Geometry check sheet. Reference: the model listing, model coordinates, mm. A direction names the side the tool comes from. Give positions to 0.01 mm unless a question says otherwise; leave off trailing zeros. Write each loop counter-clockwise with the first axis right and the second up, starting at its lowest first coordinate (ties: lowest second). Pieces come first, ordered by that corner, then holes. Notation, with made-up numbers: M 18,-19.75 L 73,-19.75 A20 ccw 73,7.25 Z; hole C 69,44 d7. An arc over 180 degrees is marked long. Write each question's results on one line, items separated by ' | '.
```python
from build123d import *

# Parameters (mm, degrees)
SKETCH1_W           = 64
SKETCH1_H           = 45
BOSS_EXTRUDE1_DEPTH = 34
SKETCH2_R           = 10.75
CUT_EXTRUDE1_DEPTH  = 6
CUT_EXTRUDE2_START  = -2
SKETCH3_W           = 60
SKETCH3_H           = 41
CUT_EXTRUDE2_DEPTH  = 27
SKETCH4_W           = 60
SKETCH4_H           = 30
CUT_EXTRUDE3_DEPTH  = 43
SKETCH5_W           = 20
SKETCH5_H           = 2
CUT_EXTRUDE4_DEPTH  = 27
BOSS_EXTRUDE2_START = 2
BOSS_EXTRUDE2_DEPTH = 5
BOSS_EXTRUDE3_START = -7
BOSS_EXTRUDE3_DEPTH = 5
SKETCH10_W          = 15.255500618
SKETCH10_H          = 37
CUT_EXTRUDE5_DEPTH  = 2


with BuildPart() as part:
    # Sketch1 → Boss-Extrude1 (new body)
    with BuildSketch(Plane.XY):
        with Locations((1.653781513, -3.994957983)):
            Rectangle(SKETCH1_W, SKETCH1_H)
    extrude(amount=BOSS_EXTRUDE1_DEPTH)

    # Sketch2 → Cut-Extrude1 (cut)
    with BuildSketch(Plane.XY.offset(34)):
        with Locations((-11.346218487, -11.494957983)):
            Circle(SKETCH2_R)
    extrude(amount=-CUT_EXTRUDE1_DEPTH, mode=Mode.SUBTRACT)

    # Sketch3 → Cut-Extrude2 (cut)
    with BuildSketch(Plane.XY.offset(34).offset(CUT_EXTRUDE2_START)):
        with Locations((1.653781513, -3.994957983)):
            Rectangle(SKETCH3_W, SKETCH3_H)
    extrude(amount=-CUT_EXTRUDE2_DEPTH, mode=Mode.SUBTRACT)

    # Sketch4 → Cut-Extrude3 (cut)
    with BuildSketch(Plane(origin=(0, 18.505042017, 0), x_dir=(1, 0, 0), z_dir=(0, 1, 0))):
        with Locations((1.653781513, -17)):
            Rectangle(SKETCH4_W, SKETCH4_H)
    extrude(amount=-CUT_EXTRUDE3_DEPTH, mode=Mode.SUBTRACT)

    # Sketch5 → Cut-Extrude4 (cut)
    with BuildSketch(Plane(origin=(0, 18.505042017, 0), x_dir=(1, 0, 0), z_dir=(0, 1, 0))):
        with Locations((-11.346218487, -33)):
            Rectangle(SKETCH5_W, SKETCH5_H)
    extrude(amount=-CUT_EXTRUDE4_DEPTH, mode=Mode.SUBTRACT)

    # Sketch7 → Boss-Extrude2 (add)
    with BuildSketch(Plane(origin=(0, 0, 0), x_dir=(0, 0, -1), z_dir=(1, 0, 0)).offset(BOSS_EXTRUDE2_START)):
        with BuildLine():
            Line((0, 7.999642933), (15, 7.999642933))
            ThreePointArc((15, 7.999642933), (25, -2.000357067), (15, -12.000357067))
            Line((15, -12.000357067), (0, -12.000357067))
            Line((0, -12.000357067), (0, 7.999642933))
        make_face()
    extrude(amount=BOSS_EXTRUDE2_DEPTH)

    # Sketch8 → Boss-Extrude3 (add)
    with BuildSketch(Plane(origin=(0, 0, 0), x_dir=(0, 0, -1), z_dir=(1, 0, 0)).offset(BOSS_EXTRUDE3_START)):
        with BuildLine():
            Line((0, -12.000357067), (0, 7.999642933))
            Line((0, 7.999642933), (15, 7.999642933))
            ThreePointArc((15, 7.999642933), (25, -2.000357067), (15, -12.000357067))
            Line((15, -12.000357067), (0, -12.000357067))
        make_face()
    extrude(amount=BOSS_EXTRUDE3_DEPTH)

    # Sketch10 → Cut-Extrude5 (cut)
    with BuildSketch(Plane.ZY.offset(30.346218487)):
        with Locations((9.627750309, 0.005042017)):
            Rectangle(SKETCH10_W, SKETCH10_H)
    extrude(amount=-CUT_EXTRUDE5_DEPTH, mode=Mode.SUBTRACT)


solid = part.part
```
Q1. Access from +Z, -Z, +X, -X, +Y, -Y to the whole of each face (thin tool, end or side, straight path). Record for faces 1 (the face through (2, -2, -13)), 2 (the face through (-21.346, 6, 33)), 3 (the face through (4, 8, -7)).
Answer key:
face 1: -Z, +Y, -Y | face 2: +Z, +Y | face 3: -Z, +X, -X, +Y
Q2. Section check B-B (x = 19). Enter the section's corners in (y, z), then the cut area to 3 significant figures.
Answer key:
outline: M -26.49,0 L 18.51,0 L 18.51,2 L -24.49,2 L -24.49,32 L 18.51,32 L 18.51,34 L -26.49,34 Z | area: 240 mm2
Q3. Release check for a two-part mould opening along Y. For faces 4 (the face through (-5, -12, -8)), 5 (the face through (-29, -18.495, 10)), 6 (the face through (-11.64, -22.24, 33.01)), 7 (the face through (31.654, -3, 17)) record: released by +Y, released by -Y, zero draft, split by the parting line, or undercut.
Answer key:
face 4: released by -Y | face 5: released by +Y | face 6: undercut | face 7: zero draft
Q4. Depth check by flat-ended pin: P1, Ø15, axis at x = -9, z = 14, coming from the +Y side; P2, Ø22.5, axis at x = 16.5, y = 6.5, coming from the -Z side; P3, Ø1.5, axis at x = 5, z = -5, coming from the -Y side. Enter the tip coordinate at first touch or a pass-through.
Answer key:
P1: stops at y = -24.49 | P2: stops at z = -24.69 | P3: stops at y = -12
Q5. Section check D-D (z = 21.5). Enter the section's corners in (x, y).
Answer key:
outline: M -30.35,-26.49 L 33.65,-26.49 L 33.65,18.51 L 31.65,18.51 L 31.65,-24.49 L -28.35,-24.49 L -28.35,18.51 L -30.35,18.51 Z
Q6. Material ranges on probe 1 along Z at (x, y) = (31, 11); probe 2 along X at (y, z) = (-7.5, -5); probe 3 along X at (y, z) = (-13, 27.5), recorded low to high. Write a range as [from, to].
Answer key:
probe 1: z = [0, 2], [32, 34] | probe 2: x = [-7, -2], [2, 7] | probe 3: x = [-30.35, -28.35], [31.65, 33.65]
Q7. Section check A-A (z = -13). Enter the section's corners in (x, y), then the cut area to 3 significant figures.
Answer key:
outline: M -7,-12 L -2,-12 L -2,8 L -7,8 Z; M 2,-12 L 7,-12 L 7,8 L 2,8 Z | area: 200 mm2
Q8. Section check C-C (y = 4). Enter the section's corners in (x, z), then the cut area to 3 significant figures.
Answer key:
outline: M -30.35,0 L -7,0 L -7,-23 L -2,-23 L -2,0 L 2,0 L 2,-23 L 7,-23 L 7,0 L 33.65,0 L 33.65,34 L -1.35,34 L -1.35,32 L 31.65,32 L 31.65,2 L -30.35,2 Z; M -30.35,17.26 L -28.35,17.26 L -28.35,32 L -21.35,32 L -21.35,34 L -30.35,34 Z | area: 535 mm2
